Build history of the part. All positions in model axes, mm. A direction names the side the tool comes from. Give positions to 0.01 mm unless a question says otherwise; leave off trailing zeros. Order: outer loops, then holes, each group sorted by start corner. A loop starts at its lowest first (then second) coordinate and runs counter-clockwise, first axis right, second up. Notation, with made-up numbers: M 20.5,31.25 L 67.5,31.25 A22 ccw 67.5,44.25 Z; hole C -23.75,-32 d10. An arc over 180 degrees is marked long. One line per item, written item: value. Start each with the question number.
from build123d import *

# Parameters (mm, degrees)
CUT_EXTRUDE1_DEPTH = 5
SKETCH3_R          = 8.5
CUT_EXTRUDE2_DEPTH = 5
SKETCH5_R          = 9.5
CUT_EXTRUDE3_DEPTH = 3
CHAMFER1_SIZE      = 1


with BuildPart() as part:
    # Sketch1 → Revolve2 (revolve)
    with BuildSketch(Plane.XY, mode=Mode.PRIVATE) as revolve2_sk:
        with BuildLine():
            Line((0, -13.216216216), (0, 58.773783784))
            Line((0, 58.773783784), (-13, 58.773783784))
            Line((-13, 58.773783784), (-13, 40.773783784))
            Line((-13, 40.773783784), (-11.5, 38.273783784))
            ThreePointArc((-11.5, 38.273783784), (-10.687594514, 35.99246344), (-8.5, 34.953783784))
            ThreePointArc((-8.5, 34.953783784), (-5.234654729, 17.897867779), (-8, 0.753783784))
            ThreePointArc((-8, 0.753783784), (-9.414213562, 0.167997346), (-10, -1.246216216))
            Line((-10, -1.246216216), (-10, -2.246216216))
            ThreePointArc((-10, -2.246216216), (-13.688325627, -5.999334736), (-13, -11.216216216))
            Line((-13, -11.216216216), (-15, -13.216216216))
            Line((-15, -13.216216216), (0, -13.216216216))
        make_face()
    revolve(revolve2_sk.sketch.rotate(Axis((0, 81.004684333, 0), (0, -1, 0)), 270), axis=Axis((0, 81.004684333, 0), (0, -1, 0)))

    # Sketch2 → Cut-Extrude1 (cut)
    with BuildSketch(Plane(origin=(0, 58.773783784, 0), x_dir=(1, 0, 0), z_dir=(0, 1, 0))):
        with BuildLine():
            Line((-3.5, 7.745966692), (-3.5, 12.519984026))
            ThreePointArc((-3.5, 12.519984026), (-9.192388155, 9.192388155), (-12.519984026, 3.5))
            Line((-12.519984026, 3.5), (-7.745966692, 3.5))
            ThreePointArc((-7.745966692, 3.5), (-6.01040764, 6.01040764), (-3.5, 7.745966692))
        make_face()
        with BuildLine():
            ThreePointArc((-12.519984026, -3.5), (-9.192388155, -9.192388155), (-3.5, -12.519984026))
            Line((-3.5, -12.519984026), (-3.5, -7.745966692))
            ThreePointArc((-3.5, -7.745966692), (-6.01040764, -6.01040764), (-7.745966692, -3.5))
            Line((-7.745966692, -3.5), (-12.519984026, -3.5))
        make_face()
        with BuildLine():
            ThreePointArc((3.5, -12.519984026), (9.192388155, -9.192388155), (12.519984026, -3.5))
            Line((12.519984026, -3.5), (7.745966692, -3.5))
            ThreePointArc((7.745966692, -3.5), (6.01040764, -6.01040764), (3.5, -7.745966692))
            Line((3.5, -7.745966692), (3.5, -12.519984026))
        make_face()
        with BuildLine():
            ThreePointArc((3.5, 7.745966692), (6.01040764, 6.01040764), (7.745966692, 3.5))
            Line((7.745966692, 3.5), (12.519984026, 3.5))
            ThreePointArc((12.519984026, 3.5), (9.192388155, 9.192388155), (3.5, 12.519984026))
            Line((3.5, 12.519984026), (3.5, 7.745966692))
        make_face()
    extrude(amount=-CUT_EXTRUDE1_DEPTH, mode=Mode.SUBTRACT)

    # Sketch3 → Cut-Extrude2 (cut)
    with BuildSketch(Plane(origin=(0, 58.773783784, 0), x_dir=(1, 0, 0), z_dir=(0, 1, 0))):
        Circle(SKETCH3_R)
    extrude(amount=-CUT_EXTRUDE2_DEPTH, mode=Mode.SUBTRACT)

    # Sketch5 → Cut-Extrude3 (cut)
    with BuildSketch(Plane(origin=(0, 53.773783784, 0), x_dir=(1, 0, 0), z_dir=(0, 1, 0))):
        with Locations(Location((0, 0, 0), (0, 0, 270))):
            Circle(SKETCH5_R)
    extrude(amount=-CUT_EXTRUDE3_DEPTH, mode=Mode.SUBTRACT)

    # Chamfer1
    chamfer1_edges = [part.edges().sort_by_distance(p)[0] for p in [
        (13, 58.773783784, 0),
        (0, 58.773783784, -13),
        (-13, 58.773783784, 0),
        (1.766381565, 58.773783784, 12.879436951),
        (8.5, 58.773783784, 0),
        (0, 58.773783784, -8.5),
        (-8.5, 58.773783784, 0),
        (0, 58.773783784, 8.5),
    ]]
    chamfer(chamfer1_edges, length=CHAMFER1_SIZE)


solid = part.part
1) Slice it at D-D (y = 1.5). List the corners of the cut face in (x, z), plus the area to 3 significant figures.
2) Pull direction Z, two halves, no side cores. Call faces 1 (the flat face through (0, 53.774, 9)), 2 (the conical face through (0.051, 58.378, 12.396)), 3 (the flat face through (8, 53.774, -8)): pulls with the +Z half, pulls with the -Z half, needs draft (parallel to the pull), parting line crosses it, or undercut.
3) Drill centre lines: line 1 (X direction, y = 52.05, z = 0); line 2 (Y direction, x = 9, z = -9); line 3 (X direction, y = 55.5, z = -9.5). Where is each one in solid material? Low to high.
4) Slice it at C-C (y = 47). List the corners of the cut face in (x, z).
5) Drop flat-ended pins along their axis: P1, Ø4, axis at x = -6.5, y = 48.5, coming from the +Z side; P2, Ø2.5, axis at x = 6, z = -7, coming from the +Y side; P3, Ø1.4, axis at x = -10.5, y = 55.5, coming from the +Z side. Give the stop position or say it passes through.
6) Tool access for faces 4 (the cylindrical face through (0.1, 55.8, -8.5)), 5 (the flat face through (-3.5, 56, -10)), 6 (the flat face through (0, 50.774, 0)): list every direction of +Z, -Z, +X, -X, +Y, -Y with a clear straight run to the whole face (end or side of a thin tool).
Results list:
1. outline: C 0,0 d15.49
1. area: 189 mm²
2. face 1: undercut
2. face 2: pulls with the +Z half
2. face 3: needs draft
3. line 1: x = -13 to -9.5, 9.5 to 13
3. line 2: y = -13.22 to -4.21, 40.32 to 53.77
3. line 3: x = -3.5 to 3.5
4. outline: C 0,0 d26
5. P1: stops at z = 12.2
5. P2: stops at y = 53.77
5. P3: stops at z = 3.5
6. face 4: +Y
6. face 5: +Z, -Z, -X, +Y
6. face 6: none
